For this review, take the finished solid that the model builds, in its own axes (mm). A direction names the side the tool comes from. Coordinates: 2 decimals unless noted, no trailing zeros. Loops run counter-clockwise (first coordinate to the right, second up) from the corner with the lowest first, then second, coordinate; pieces in that order, holes last. Notation, with made-up numbers: (77.5, 59.5) -> (91.5, 59.5) arc R26 cw to (91.5, 76.5) -> close; hole circle Ø2 at (0.5, 74). An arc over 180 degrees is marked (long way). One line per item, written item: value.
from build123d import *

# Parameters (mm, degrees)
EXTRUDE_1_DEPTH = 9
EXTRUDE_2_DEPTH = 3
SKETCH_1_5_R    = 4.5
SKETCH_1_5_R_2  = 2.5
EXTRUDE_3_DEPTH = 1.5
SKETCH_1_7_R    = 3.5
SKETCH_1_7_R_2  = 2.25
EXTRUDE_4_DEPTH = 1
SKETCH_1_8_R    = 14
EXTRUDE_5_DEPTH = 19
SKETCH_1_9_W    = 2.5
SKETCH_1_9_H    = 14.5
EXTRUDE_6_DEPTH = 16.5
EXTRUDE_START   = -3.5
EXTRUDE_7_DEPTH = 12.5


with BuildPart() as part:
    # Sketch 1 → Extrude 1 (new body)
    with BuildSketch(Plane(origin=(0, 0, 0), x_dir=(1, 0, 0), z_dir=(0, 1, 0))):
        with BuildLine():
            ThreePointArc((9.5, 2), (8, 2.5), (6.5, 2))
            Line((6.5, 2), (6.5, -2))
            ThreePointArc((6.5, -2), (8, -2.5), (9.5, -2))
            Line((9.5, -2), (9.5, 2))
        make_face()
    extrude(amount=EXTRUDE_1_DEPTH)

    # Sketch 1_4 → Extrude 2 (add)
    with BuildSketch(Plane(origin=(0, 0, 0), x_dir=(1, 0, 0), z_dir=(0, 1, 0))):
        with BuildLine():
            Line((6.5, -2), (6.5, 2))
            ThreePointArc((6.5, 2), (5.5, 0), (6.5, -2))
        make_face()
        with BuildLine():
            ThreePointArc((10.5, 0), (10.236067977, 1.118033989), (9.5, 2))
            Line((9.5, 2), (9.5, -2))
            ThreePointArc((9.5, -2), (10.236067977, -1.118033989), (10.5, 0))
        make_face()
    extrude(amount=EXTRUDE_2_DEPTH)

    # Sketch 1_5 → Extrude 3 (add)
    with BuildSketch(Plane(origin=(0, 0, 0), x_dir=(1, 0, 0), z_dir=(0, 1, 0))):
        with Locations(Location((8, 0, 0), (0, 0, 270))):
            Circle(SKETCH_1_5_R)
        with Locations(Location((8, 0, 0), (0, 0, 126.869897646))):
            Circle(SKETCH_1_5_R_2, mode=Mode.SUBTRACT)
    extrude(amount=EXTRUDE_3_DEPTH)



with BuildPart() as body_2:
    # Sketch 1_7 → Extrude 4 (new body)
    # profile 1 of 6: a face of its own
    with BuildSketch(Plane(origin=(0, 0, 0), x_dir=(1, 0, 0), z_dir=(0, 1, 0))):
        with BuildLine():
            Line((-3.5, 17.5), (-3.5, 13.555441712))
            ThreePointArc((-3.5, 13.555441712), (-1.764060095, 13.888415748), (0, 14))
            ThreePointArc((0, 14), (-2.474873734, 15.025126266), (-3.5, 17.5))
        make_face()
    # profile 2 of 6: a face of its own
    with BuildSketch(Plane(origin=(0, 0, 0), x_dir=(1, 0, 0), z_dir=(0, 1, 0))):
        with Locations((0, 17.5)):
            Circle(SKETCH_1_7_R)
        with Locations(Location((0, 17.5, 0), (0, 0, 270))):
            Circle(SKETCH_1_7_R_2, mode=Mode.SUBTRACT)
    # profile 3 of 6: a face of its own
    with BuildSketch(Plane(origin=(0, 0, 0), x_dir=(1, 0, 0), z_dir=(0, 1, 0))):
        with BuildLine():
            ThreePointArc((3.5, 17.5), (2.474873734, 15.025126266), (0, 14))
            ThreePointArc((0, 14), (1.764060095, 13.888415748), (3.5, 13.555441712))
            Line((3.5, 13.555441712), (3.5, 17.5))
        make_face()
    # profile 4 of 6: a face of its own
    with BuildSketch(Plane(origin=(0, 0, 0), x_dir=(1, 0, 0), z_dir=(0, 1, 0))):
        with BuildLine():
            ThreePointArc((3.5, -13.555441712), (1.764060095, -13.888415748), (0, -14))
            ThreePointArc((0, -14), (2.474873734, -15.025126266), (3.5, -17.5))
            Line((3.5, -17.5), (3.5, -13.555441712))
        make_face()
    # profile 5 of 6: a face of its own
    with BuildSketch(Plane(origin=(0, 0, 0), x_dir=(1, 0, 0), z_dir=(0, 1, 0))):
        with Locations((0, -17.5)):
            Circle(SKETCH_1_7_R)
        with Locations(Location((0, -17.5, 0), (0, 0, 270))):
            Circle(SKETCH_1_7_R_2, mode=Mode.SUBTRACT)
    # profile 6 of 6: a face of its own
    with BuildSketch(Plane(origin=(0, 0, 0), x_dir=(1, 0, 0), z_dir=(0, 1, 0))):
        with BuildLine():
            ThreePointArc((0, -14), (-1.764060095, -13.888415748), (-3.5, -13.555441712))
            Line((-3.5, -13.555441712), (-3.5, -17.5))
            ThreePointArc((-3.5, -17.5), (-2.474873734, -15.025126266), (0, -14))
        make_face()
    extrude(amount=-EXTRUDE_4_DEPTH)


with BuildPart() as part_1:
    add(part.part)

    add(body_2.part)  # Extrude 5 merges body 2
    # Sketch 1_8 → Extrude 5 (add)
    with BuildSketch(Plane(origin=(0, 0, 0), x_dir=(1, 0, 0), z_dir=(0, 1, 0))):
        with Locations(Location((0, 0, 0), (0, 0, 270))):
            Circle(SKETCH_1_8_R)
    extrude(amount=-EXTRUDE_5_DEPTH)

    # Sketch 1_9 → Extrude 6 (add)
    with BuildSketch(Plane(origin=(0, 0, 0), x_dir=(1, 0, 0), z_dir=(0, 1, 0))):
        with Locations((-15.75, 0)):
            Rectangle(SKETCH_1_9_W, SKETCH_1_9_H)
        with BuildLine():
            ThreePointArc((-11.976539567, -7.25), (-14, 0), (-11.976539567, 7.25))
            Line((-11.976539567, 7.25), (-14.5, 7.25))
            Line((-14.5, 7.25), (-14.5, -7.25))
            Line((-14.5, -7.25), (-11.976539567, -7.25))
        make_face()
    extrude(amount=-EXTRUDE_6_DEPTH)

    # Sketch 1_10 → Extrude 7 (add)
    with BuildSketch(Plane(origin=(0, 0, 0), x_dir=(1, 0, 0), z_dir=(0, 1, 0)).offset(EXTRUDE_START)):
        with BuildLine():
            ThreePointArc((-11.976539567, 7.25), (-11.477174409, 8.017135871), (-10.928746497, 8.75))
            Line((-10.928746497, 8.75), (-14.5, 8.75))
            Line((-14.5, 8.75), (-14.5, 7.25))
            Line((-14.5, 7.25), (-11.976539567, 7.25))
        make_face()
        with BuildLine():
            ThreePointArc((-10.928746497, -8.75), (-11.477174409, -8.017135871), (-11.976539567, -7.25))
            Line((-11.976539567, -7.25), (-14.5, -7.25))
            Line((-14.5, -7.25), (-14.5, -8.75))
            Line((-14.5, -8.75), (-10.928746497, -8.75))
        make_face()
    extrude(amount=-EXTRUDE_7_DEPTH)


solid = part_1.part
1. Insertion check: pin 1 Ø4 at (x, y) = (-12.5, -11.5) entering from -Z; pin 2 Ø0.8 at (y, z) = (-0.5, 16.5) entering from -X; pin 3 Ø15.5 at (x, z) = (1, -8.5) entering from +Y; pin 4 Ø12 at (y, z) = (-5.5, -4.5) entering from +X. Each pin has a flat end and moves straight along its axis. Give the tip position at first contact, or say it passes through.
Return value:
pin 1: stops at z = -9.26
pin 2: stops at x = -3.5
pin 3: stops at y = 1.5
pin 4: stops at x = 14
2. Take a section at C-C, the plane y = -5.25. Give the boundary of the cut face in (x, z), and give its area (3 significant figures).
Return value:
outline: (-17, -7.25) -> (-14.5, -7.25) -> (-14.5, -8.75) -> (-10.93, -8.75) arc R14 ccw (long way) to (-10.93, 8.75) -> (-14.5, 8.75) -> (-14.5, 7.25) -> (-17, 7.25) -> close
area: 678 mm2
3. The part is to be moulded in two halves that separate along Z. For faces 5 (the cylindrical face through (0.676, -0.493, 19.646)), 6 (the flat face through (3.5, -0.5, 15.6)), 7 (the flat face through (-13, -10, -8.75)), 8 (the cylindrical face through (0.676, -0.493, -15.354)), say which applies: pulls with the +Z half, pulls with the -Z half, needs draft (parallel to the pull), parting line crosses it, or undercut.
Return value:
face 5: undercut
face 6: needs draft
face 7: pulls with the -Z half
face 8: undercut
4. For faces 1 (the flat face through (-13, -16, 8)), 2 (the flat face through (-3.5, -0.5, 15.5)), 3 (the flat face through (10, 3, 0)), 4 (the flat face through (-13, -3.5, -8)), list the 3-axis set-ups (+Z, -Z, +X, -X, +Y, -Y) from which the entire face can be reached by the end or side of a thin tool; tool diameter is ignored.
Return value:
face 1: +Z, -X, -Y
face 2: +Z, -X, +Y, -Y
face 3: +Z, -Z, +X, +Y
face 4: -Z, -X, +Y
5. Take a section at A-A, the plane x = 0.5. Give the boundary of the cut face in (y, z).
Return value:
outline: (-19, -13.99) -> (-1, -13.99) -> (-1, -15.31) -> (0, -15.31) -> (0, 15.31) -> (-1, 15.31) -> (-1, 13.99) -> (-19, 13.99) -> close; (-1, -20.96) -> (0, -20.96) -> (0, -19.69) -> (-1, -19.69) -> close; (-1, 19.69) -> (0, 19.69) -> (0, 20.96) -> (-1, 20.96) -> close
6. To check wall thickness, follow probe 1 along X at (y, z) = (-0.15, -17.5); probe 2 along Y at (x, z) = (-1, 1); probe 3 along X at (y, z) = (-7.75, -10). State the ranges of each line that lie inside material, in increasing order. Write a range as from..to.
Return value:
probe 1: x = -3.5..-2.25, 2.25..3.5
probe 2: y = -19..0
probe 3: x = -9.8..9.8
7. Take a section at B-B, the plane z = 0. Give the boundary of the cut face in (x, y).
Return value:
outline: (-17, -16.5) -> (-14, -16.5) -> (-14, -19) -> (14, -19) -> (14, 0) -> (12.5, 0) -> (12.5, 1.5) -> (10.5, 1.5) -> (10.5, 3) -> (9.5, 3) -> (9.5, 9) -> (6.5, 9) -> (6.5, 3) -> (5.5, 3) -> (5.5, 1.5) -> (3.5, 1.5) -> (3.5, 0) -> (-17, 0) -> close
8. Take a section at D-D, the plane z = -16.5. Give the boundary of the cut face in (x, y), and give its area (3 significant figures).
Return value:
outline: (-3.5, -1) -> (-2.02, -1) -> (-2.02, 0) -> (-3.5, 0) -> close; (2.02, -1) -> (3.5, -1) -> (3.5, 0) -> (2.02, 0) -> close
area: 2.97 mm2
